from build123d import *

# Parameters (mm, degrees)
BOSS_EXTRUDE1_DEPTH     = 32.5
SHELL4_START            = -27.5
SHELL4_DEPTH            = 55
CUT_EXTRUDE2_DEPTH      = 21
CUT_EXTRUDE2_DEPTH_BACK = 20
SKETCH4_W               = 55
SKETCH4_H               = 18
CHAMFER18_START         = -24
CHAMFER18_OUTLINE_W     = 10
CHAMFER18_OUTLINE_H     = 57
CHAMFER18_DEPTH         = 4.554563517
CHAMFER36_START         = 19.445436483
CHAMFER36_OUTLINE_W     = 10
CHAMFER36_OUTLINE_H     = 57
CHAMFER36_DEPTH         = 4.554563517
SKETCH8_R               = 2.6
SKETCH8_R_2             = 1.75
SKETCH8_R_3             = 5
SKETCH8_R_4             = 3.5
SKETCH8_R_5             = 1.25
CUT_EXTRUDE4_DEPTH      = 185
CUT_EXTRUDE6_DEPTH      = 4.5
CUT_EXTRUDE8_DEPTH      = 17
CUT_EXTRUDE8_DEPTH_BACK = 5.1
SKETCH13_R              = 1.5
SKETCH14_R              = 1.75
BOSS_EXTRUDE2_DEPTH     = 5


with BuildPart() as part:
    # Sketch3 → Boss-Extrude1 (new, symmetric)
    with BuildSketch(Plane(origin=(0, 0, 0), x_dir=(0, 0, -1), z_dir=(1, 0, 0))):
        with BuildLine():
            Line((0, 50), (-20.96, 71.073578053))
            ThreePointArc((-20.96, 71.073578053), (-44.01947273, 71.403830624), (-44.885431169, 48.358256964))
            Line((-44.885431169, 48.358256964), (-21, 22))
            Line((-21, 22), (-21, 0))
            Line((-21, 0), (0, 0))
            Line((0, 0), (0, 50))
        make_face()
    extrude(amount=BOSS_EXTRUDE1_DEPTH, both=True)

    # Shell4: read off the stored shape, not the designer's step
    # Shell4 outline → Shell4 (cut)
    with BuildSketch(Plane.YZ.offset(SHELL4_START)):
        with BuildLine():
            Line((51.715719855, 41.180374768), (48.358256964, 44.885431169))
            Line((48.358256964, 44.885431169), (22, 21))
            Line((22, 21), (5, 21))
            Line((5, 21), (5, 0))
            Line((5, 0), (50, 0))
            Line((50, 0), (71.073578053, 20.96))
            Line((71.073578053, 20.96), (67.547610311, 24.505074257))
            ThreePointArc((67.547610311, 24.505074257), (67.777786345, 40.576827978), (51.715719855, 41.180374768))
        make_face()
    extrude(amount=SHELL4_DEPTH, mode=Mode.SUBTRACT)

    # Sketch4 → Cut-Extrude2 (cut, two sides: drawn at the far end of the back side and taken through both)
    with BuildSketch(Plane.XZ.offset(-CUT_EXTRUDE2_DEPTH_BACK)):
        with Locations((0, 9)):
            Rectangle(SKETCH4_W, SKETCH4_H)
    extrude(amount=CUT_EXTRUDE2_DEPTH + CUT_EXTRUDE2_DEPTH_BACK, mode=Mode.SUBTRACT)

    # Chamfer18: read off the stored shape, not the designer's step
    # Chamfer18 outline → Chamfer18 (cut)
    with BuildSketch(Plane(origin=(0, 0, 0), x_dir=(0.707106781186548, 0, -0.707106781186547), z_dir=(0.707106781186547, 0, 0.707106781186548)).offset(CHAMFER18_START)):
        with Locations((-23, 28.5)):
            Rectangle(CHAMFER18_OUTLINE_W, CHAMFER18_OUTLINE_H)
    extrude(amount=CHAMFER18_DEPTH, mode=Mode.SUBTRACT)

    # Chamfer36: read off the stored shape, not the designer's step
    # Chamfer36 outline → Chamfer36 (cut)
    with BuildSketch(Plane(origin=(0, 0, 0), x_dir=(0.707106781186548, 0, 0.707106781186547), z_dir=(0.707106781186547, 0, -0.707106781186548)).offset(CHAMFER36_START)):
        with Locations((23, -28.5)):
            Rectangle(CHAMFER36_OUTLINE_W, CHAMFER36_OUTLINE_H)
    extrude(amount=CHAMFER36_DEPTH, mode=Mode.SUBTRACT)

    # Sketch8 → Cut-Extrude4 (cut)
    with BuildSketch(Plane.ZY.offset(33.5)):
        with Locations(Location((5, 10, 0), (0, 0, 270))):
            Circle(SKETCH8_R)
        with Locations(Location((14, 10, 0), (0, 0, 180))):
            Circle(SKETCH8_R_2)
        with Locations(Location((14, 16, 0), (0, 0, 180))):
            Circle(SKETCH8_R_2)
        with Locations(Location((26.852977749, 51.641327413, 0), (0, 0, 180))):
            Circle(SKETCH8_R_3)
        with Locations(Location((10, 37.5, 0), (0, 0, 180))):
            Circle(SKETCH8_R_4)
        with Locations(Location((35.25759337, 46.292268033, 0), (0, 0, 180))):
            Circle(SKETCH8_R_5)
        with Locations(Location((23.044628786, 60.847112452, 0), (0, 0, 180))):
            Circle(SKETCH8_R_5)
    extrude(amount=-CUT_EXTRUDE4_DEPTH, mode=Mode.SUBTRACT)

    # Sketch10 → Cut-Extrude6 (cut)
    with BuildSketch(Plane.ZY.offset(34.5)):
        with BuildLine():
            ThreePointArc((16.645751311, 13), (14, 20), (11.354248689, 13))
            ThreePointArc((11.354248689, 13), (14, 6), (16.645751311, 13))
        make_face()
        with BuildLine():
            ThreePointArc((12.476565423, 49.752208932), (0.424444461, 29.465154879), (22.49612142, 37.811367076))
            ThreePointArc((22.49612142, 37.811367076), (37.960622174, 60.961747754), (12.476565423, 49.752208932))
        make_face()
    cut_extrude6 = extrude(amount=-CUT_EXTRUDE6_DEPTH, mode=Mode.SUBTRACT)

    # Mirror1: Cut-Extrude6 across plane
    add(cut_extrude6.mirror(Plane(origin=(0, 0, 0), x_dir=(0, 0, 1), z_dir=(1, 0, 0))), mode=Mode.SUBTRACT)

    # Sketch13 → Cut-Extrude8 (cut, two sides: drawn at the far end of the back side and taken through both)
    with BuildSketch(Plane.XZ.offset(-CUT_EXTRUDE8_DEPTH_BACK)):
        with Locations(Location((-30, 11.354248689, 0), (0, 0, 90))):
            Circle(SKETCH13_R)
        with Locations(Location((30, 11.354248689, 0), (0, 0, 90))):
            Circle(SKETCH13_R)
    extrude(amount=CUT_EXTRUDE8_DEPTH + CUT_EXTRUDE8_DEPTH_BACK, mode=Mode.SUBTRACT)

    # Sketch14 → Boss-Extrude2 (add)
    # profile 1 of 2: a face of its own
    with BuildSketch(Plane.XZ):
        with BuildLine():
            Line((-3.749981176, 23), (-3.749981176, 21))
            Line((-3.749981176, 21), (-11.249981176, 21))
            Line((-11.249981176, 21), (-11.249981176, 23))
            ThreePointArc((-11.249981176, 23), (-7.499981176, 26.75), (-3.749981176, 23))
        make_face()
        with Locations(Location((-7.499981176, 23, 0), (0, 0, 270))):
            Circle(SKETCH14_R, mode=Mode.SUBTRACT)
    # profile 2 of 2: a face of its own
    with BuildSketch(Plane.XZ):
        with BuildLine():
            Line((3.750018824, 23), (3.750018824, 20.96))
            Line((3.750018824, 20.96), (11.250018824, 20.96))
            Line((11.250018824, 20.96), (11.250018824, 23))
            ThreePointArc((11.250018824, 23), (7.500018824, 26.75), (3.750018824, 23))
        make_face()
        with Locations(Location((7.500018824, 23, 0), (0, 0, 270))):
            Circle(SKETCH14_R, mode=Mode.SUBTRACT)
    extrude(amount=-BOSS_EXTRUDE2_DEPTH)


solid = part.part
Can you work these out from the model? Positions are in its coordinate system, mm. A direction names the side the tool comes from. Give positions to 0.01 mm unless a question says otherwise; leave off trailing zeros. Order: outer loops, then holes, each group sorted by start corner. A loop starts at its lowest first (then second) coordinate and runs counter-clockwise, first axis right, second up. Notation, with made-up numbers: M -17,-6.75 L 22,-6.75 A31 ccw 22,31.25 Z; hole C -27.5,-27.5 d5. An arc over 180 degrees is marked long. Use one line per item in the form item = value. Start each with the question number.
Item 1: If we section it at B-B (y = 16): Write out the boundary of the cut face in (x, z).
Item 2: If we section it at C-C (z = 30.5): Write out the boundary of the cut face in (x, y), then the cut area to 3 significant figures.
Item 3: If we section it at D-D (z = 43): Write out the boundary of the cut face in (x, y).
Item 4: If I drill on line 1 along X through (y, z) = (2.25, 23); line 2 along X through (y, z) = (52, 8); line 3 along X through (y, z) = (53, 33), over which ranges is the centre line in solid material (lowest first)?
Item 5: We'd pull the mould along Y, two halves only. Please class faces 6 (the cylindrical face through (-28.768, 61.956, 22.468)), 7 (the flat face through (-29.965, 35.364, 33.11)), 8 (the cylindrical face through (-0.39, 67.95, 40.39)), 9 (the flat face through (29, 6, 21)): +Y half, -Y half, draft (parallel to the pull), parting line (faces both ways), or undercut.
Item 6: For faces 1 (the flat face through (-3.75, 2, 22)), 2 (the cylindrical face through (28.986, 2.586, 10.249)), 3 (the cylindrical face through (31.268, 49.906, 8.473)), 4 (the cylindrical face through (-31, 6, 14)), 5 (the flat face through (-29.96, 62.73, 12.66)), which set-ups out of +Z, -Z, +X, -X, +Y, -Y let a thin tool reach every point of the face, with its end or its side?
Item 7: Will these pins go through, and if not, where does the flat tip stop? pin 1 Ø1.5 at (y, z) = (58, 21) entering from +X; pin 2 Ø8 at (x, z) = (17.5, 40) entering from -Y; pin 3 Ø1.5 at (y, z) = (60.85, 23.04) entering from +X (1 decimal); pin 4 Ø4.5 at (x, z) = (-8, 22) entering from +Y.
Outcome:
q1.outline = M -32.5,5 L -27.5,0 L -27.5,12.25 L -30,12.25 L -30,10 L -32.5,10 Z; M -32.5,18 L -30,18 L -30,15.75 L -27.5,15.75 L -27.5,21 L -32.5,21 Z; M 27.5,0 L 32.5,5 L 32.5,10 L 30,10 L 30,12.25 L 27.5,12.25 Z; M 27.5,15.75 L 30,15.75 L 30,18 L 32.5,18 L 32.5,21 L 27.5,21 Z
q2.outline = M -32.5,32.48 L -27.5,32.48 L -27.5,48.22 L -30,48.22 L -30,37.61 L -32.5,37.61 Z; M -32.5,65.68 L -30,65.68 L -30,55.06 L -27.5,55.06 L -27.5,70.73 L 27.5,70.73 L 27.5,55.06 L 30,55.06 L 30,65.68 L 32.5,65.68 L 32.5,75.8 L -32.5,75.8 Z; M 27.5,32.48 L 32.5,32.48 L 32.5,37.61 L 30,37.61 L 30,48.22 L 27.5,48.22 Z
q2.area = 537 mm2
q3.outline = M -32.5,46.28 L -27.5,46.28 L -27.5,50.07 L 27.5,50.07 L 27.5,46.28 L 32.5,46.28 L 32.5,72.3 L -32.5,72.3 Z; hole M -27.5,54.41 L 27.5,54.41 L 27.5,64.47 L -27.5,64.47 Z
q4.line_1 = -11.25 to -9.25, -5.75 to -3.75, 3.75 to 5.75, 9.25 to 11.25
q4.line_2 = -32.5 to -27.5, 27.5 to 32.5
q4.line_3 = -30 to -27.5, 27.5 to 30
q5.face_6 = undercut
q5.face_7 = -Y half
q5.face_8 = undercut
q5.face_9 = draft
q6.face_1 = +Z, -Y
q6.face_2 = -Y
q6.face_3 = +X
q6.face_4 = -X
q6.face_5 = -Z, +X, -X, +Y
q7.pin_1 = 30
q7.pin_2 = 49.16
q7.pin_3 = through
q7.pin_4 = 73.63
